The listing builds one solid part. Answer for the finished solid, in the listing's coordinates (mm). A direction names the side the tool comes from. Give positions to 0.01 mm unless a question says otherwise; leave off trailing zeros. Loops run counter-clockwise (first coordinate to the right, second up) from the corner with the lowest first, then second, coordinate; pieces in that order, holes last. Notation, with made-up numbers: M 13,7 L 43,7 A9 cw 43,15 Z; hole C -34.75,75.5 d1. An arc over 180 degrees is marked long. Return JSON: item names as keys, results as strings.
from build123d import *

# Parameters (mm, degrees)
BOSS_EXTRUDE1_DEPTH = 1.524


with BuildPart() as part:
    # Sketch1 → Boss-Extrude1 (new body)
    with BuildSketch(Plane.XY):
        with BuildLine():
            Line((-31.115654525, 85.743001786), (-31.626029854, 93.062039695))
            ThreePointArc((-31.626029854, 93.062039695), (-30.088685306, 91.89525557), (-28.45677625, 90.864873946))
            ThreePointArc((-28.45677625, 90.864873946), (-24.332080512, 90.260671192), (-21.042280839, 87.700320822))
            ThreePointArc((-21.042280839, 87.700320822), (-17.253316375, 85.808122938), (-13.994450183, 83.103228173))
            ThreePointArc((-13.994450183, 83.103228173), (-9.99101498, 81.01245123), (-6.834531764, 77.782055688))
            ThreePointArc((-6.834531764, 77.782055688), (-9.047280649, 78.959528297), (-11.434463645, 79.723764333))
            ThreePointArc((-11.434463645, 79.723764333), (-9.401311851, 74.738116942), (-8.891074145, 69.378075561))
            ThreePointArc((-8.891074145, 69.378075561), (-8.368327541, 68.796388825), (-7.866530285, 68.196536356))
            ThreePointArc((-7.866530285, 68.196536356), (-5.298466146, 67.533161121), (-3.150709885, 65.976831091))
            ThreePointArc((-3.150709885, 65.976831091), (-4.721037121, 66.188066002), (-6.291364357, 65.976831091))
            ThreePointArc((-6.291364357, 65.976831091), (-4.243849878, 61.717361935), (-3.150709885, 57.119488733))
            ThreePointArc((-3.150709885, 57.119488733), (-1.695723101, 55.731011208), (-0.531968435, 54.090727251))
            ThreePointArc((-0.531968435, 54.090727251), (-1.486021988, 54.647848886), (-2.584432422, 54.76658058))
            ThreePointArc((-2.584432422, 54.76658058), (-2.443936558, 53.294197652), (-2.174566125, 51.839862702))
            ThreePointArc((-2.174566125, 51.839862702), (-1.778406294, 50.414833592), (-1.258523697, 49.030141329))
            ThreePointArc((-1.258523697, 49.030141329), (-0.531968435, 45.93780464), (-0.893428223, 42.781893428))
            ThreePointArc((-0.893428223, 42.781893428), (0.100022048, 42.0811278), (0.742668626, 41.049129115))
            ThreePointArc((0.742668626, 41.049129115), (-0.079058418, 41.323600355), (-0.941146572, 41.409471254))
            ThreePointArc((-0.941146572, 41.409471254), (0.437078702, 34.619334125), (0.303865798, 27.692017078))
            ThreePointArc((0.303865798, 27.692017078), (1.362217268, 26.063134365), (1.940723645, 24.208761938))
            ThreePointArc((1.940723645, 24.208761938), (1.068913801, 24.887622398), (0.048705917, 25.311980504))
            ThreePointArc((0.048705917, 25.311980504), (-0.439629904, 21.681833995), (-2.339389119, 18.550165034))
            ThreePointArc((-2.339389119, 18.550165034), (-3.997880754, 22.322683164), (-6.834531764, 25.311980504))
            ThreePointArc((-6.834531764, 25.311980504), (-6.056862602, 41.475358139), (-11.434463645, 56.737761388))
            ThreePointArc((-11.434463645, 56.737761388), (-18.290136293, 65.474182448), (-17.253316375, 76.530868427))
            ThreePointArc((-17.253316375, 76.530868427), (-25.334641834, 79.406189783), (-31.115654525, 85.743001786))
        make_face()
    extrude(amount=BOSS_EXTRUDE1_DEPTH)


solid = part.part
(1) A tool of negligible diameter and unlimited length cuts with its end or side. For faces 4 (the cylindrical face through (-5.33, 67.55, 0.75)), 5 (the cylindrical face through (-1.471, 54.643, 0.751)), 6 (the cylindrical face through (-3.966, 22.274, 0.751)), from which of +Z, -Z, +X, -X, +Y, -Y can it reach the whole face along a straight path? Write none if from no direction.
Values follow:
{"face 4": "+Z, -Z, +X", "face 5": "+Z, -Z", "face 6": "+Z, -Z, -X, -Y"}
(2) Given pin 1 (3 mm diameter, centred on x = -2.5, y = 65.5, fed in from +Z), flat-ended and moving along its own axis, determine where the tip first touches the part or whether it passes through.
Values follow:
{"pin 1": "z = 1.52"}
(3) The part is cut by section A-A (z = 0.6). Determine the outline of the cut face in (x, y).
Values follow:
{"outline": "M -31.63,93.06 L -31.12,85.74 A17.7 ccw -17.25,76.53 A14.99 ccw -11.43,56.74 A42.09 cw -6.83,25.31 A12 cw -2.34,18.55 A8.96 ccw 0.05,25.31 A4.14 cw 1.94,24.21 A7.12 ccw 0.3,27.69 A31.63 ccw -0.94,41.41 A3.89 cw 0.74,41.05 A3.06 ccw -0.89,42.78 A9.26 ccw -1.26,49.03 A16.81 cw -2.58,54.77 A2.64 cw -0.53,54.09 A10.51 ccw -3.15,57.12 A22.06 ccw -6.29,65.98 A5.94 cw -3.15,65.98 A7.13 ccw -7.87,68.2 A22.06 ccw -8.89,69.38 A18.49 ccw -11.43,79.72 A14.01 cw -6.83,77.78 A14.37 ccw -13.99,83.1 A18.49 ccw -21.04,87.7 A8.17 ccw -28.46,90.86 A22.44 cw Z"}
(4) Determine the mould class of faces 1 (the cylindrical face through (0.428, 34.716, 0.751)), 2 (the cylindrical face through (-30.11, 91.91, 0.75)), 3 (the flat face through (-12, 61, 0)) for opening direction Y: released by +Y, released by -Y, zero draft, split by the parting line, or undercut.
Values follow:
{"face 1": "undercut", "face 2": "released by +Y", "face 3": "zero draft"}
(5) The part is cut by section C-C (x = -24). Determine the outline of the cut face in (y, z), and give its area (3 significant figures).
Values follow:
{"outline": "M 78.6,0 L 90.11,0 L 90.11,1.52 L 78.6,1.52 Z", "area": "17.5 mm²"}
(6) Straight lines are drawn through the part: line 1 along X through (y, z) = (69.5, 0.8); line 2 along Y through (x, z) = (-15.5, 0.45); line 3 along Y through (x, z) = (-13, 1.45). For each, find the intervals that lie inside material, in ascending order.
Values follow:
{"line 1": "-18.9 to -8.89", "line 2": "60.2 to 84.51", "line 3": "57.78 to 82.73"}
(7) The part is cut by section B-B (y = 33). Determine the outline of the cut face in (x, z), and give its area (3 significant figures).
Values follow:
{"outline": "M -5.68,0 L 0.54,0 L 0.54,1.52 L -5.68,1.52 Z", "area": "9.48 mm²"}
